```python
from build123d import *

# Parameters (mm, degrees)
SKETCH_W        = 203
SKETCH_H        = 130
SKETCH_R        = 1.75
PAD_DEPTH       = 3
SKETCH001_W     = 4
SKETCH001_H     = 10
PAD001_DEPTH    = 10
SKETCH002_R     = 1.75
SKETCH002_W     = 95
SKETCH002_H     = 4
POCKET_DEPTH    = 225
SKETCH003_R     = 1.75
POCKET001_DEPTH = 200.001


with BuildPart() as part:
    # Sketch → Pad (new body)
    with BuildSketch(Plane.XY):
        with Locations((101.5, 65)):
            Rectangle(SKETCH_W, SKETCH_H)
        with Locations((22, 126.5)):
            Circle(SKETCH_R, mode=Mode.SUBTRACT)
        with Locations((100, 126.5)):
            Circle(SKETCH_R, mode=Mode.SUBTRACT)
        with Locations((178, 126.5)):
            Circle(SKETCH_R, mode=Mode.SUBTRACT)
        with Locations((22, 3.5)):
            Circle(SKETCH_R, mode=Mode.SUBTRACT)
        with Locations((100, 3.5)):
            Circle(SKETCH_R, mode=Mode.SUBTRACT)
        with Locations((178, 3.5)):
            Circle(SKETCH_R, mode=Mode.SUBTRACT)
        with BuildLine():
            ThreePointArc((15, 106.75), (13.25, 105), (15, 103.25))
            Line((15, 103.25), (95, 103.25))
            ThreePointArc((95, 103.25), (96.75, 105), (95, 106.75))
            Line((15, 106.75), (95, 106.75))
        make_face(mode=Mode.SUBTRACT)
        with BuildLine():
            ThreePointArc((14.985188, 96.750011), (13.235188, 95.000011), (14.985188, 93.250011))
            Line((14.985188, 93.250011), (94.985188, 93.250011))
            ThreePointArc((94.985188, 93.250011), (96.735188, 95.000011), (94.985188, 96.750011))
            Line((14.985188, 96.750011), (94.985188, 96.750011))
        make_face(mode=Mode.SUBTRACT)
        with BuildLine():
            ThreePointArc((14.970376, 86.750022), (13.220376, 85.000022), (14.970376, 83.250022))
            Line((14.970376, 83.250022), (94.970376, 83.250022))
            ThreePointArc((94.970376, 83.250022), (96.720376, 85.000022), (94.970376, 86.750022))
            Line((14.970376, 86.750022), (94.970376, 86.750022))
        make_face(mode=Mode.SUBTRACT)
        with BuildLine():
            ThreePointArc((14.955564, 76.750033), (13.205564, 75.000033), (14.955564, 73.250033))
            Line((14.955564, 73.250033), (94.955564, 73.250033))
            ThreePointArc((94.955564, 73.250033), (96.705564, 75.000033), (94.955564, 76.750033))
            Line((14.955564, 76.750033), (94.955564, 76.750033))
        make_face(mode=Mode.SUBTRACT)
        with BuildLine():
            ThreePointArc((14.940752, 66.750044), (13.190752, 65.000044), (14.940752, 63.250044))
            Line((14.940752, 63.250044), (94.940752, 63.250044))
            ThreePointArc((94.940752, 63.250044), (96.690752, 65.000044), (94.940752, 66.750044))
            Line((14.940752, 66.750044), (94.940752, 66.750044))
        make_face(mode=Mode.SUBTRACT)
    extrude(amount=-PAD_DEPTH)

    # Sketch001 (on DatumPlane) → Pad001 (join)
    with BuildSketch(Plane.XY.offset(-3)):
        with Locations((198, 125)):
            Rectangle(SKETCH001_W, SKETCH001_H)
        with Locations((5, 125)):
            Rectangle(SKETCH001_W, SKETCH001_H)
    extrude(amount=-PAD001_DEPTH)

    # Sketch002 → Pocket (cut)
    with BuildSketch(Plane.YZ.offset(107)):
        with Locations((-51, 7)):
            Circle(SKETCH002_R)
        with Locations((61, 7)):
            Circle(SKETCH002_R)
        with Locations((7.5, 11)):
            Rectangle(SKETCH002_W, SKETCH002_H)
    extrude(amount=-POCKET_DEPTH, mode=Mode.SUBTRACT)

    # Sketch003 (on DatumPlane) → Pocket001 (cut, through all)
    with BuildSketch(Plane.YZ.offset(3)):
        with Locations((126.5, -6.5)):
            Circle(SKETCH003_R)
    extrude(amount=POCKET001_DEPTH, mode=Mode.SUBTRACT)


solid = part.part
```
Check sheet for the modelled part. Datum: model origin and axes. Units: mm. A direction names the side the tool comes from. Coordinates: 2 decimals unless noted, no trailing zeros. Order: outer loops, then holes, each group sorted by start corner. A loop starts at its lowest first (then second) coordinate and runs counter-clockwise, first axis right, second up. Notation, with made-up numbers: M -33.75,68.5 L -18.75,68.5 A25 cw -18.75,100.5 Z; hole C 56,74 d8. An arc over 180 degrees is marked long. One line per question, with ' | ' between items. Start each with the question number.
Item 1: Mould release check, pull along X, two halves, no side actions. Record for faces 1 (the flat face through (198, 125, -13)), 2 (the flat face through (7, 125, -8)), 3 (the flat face through (3, 125, -8)): pulls with the +X half, pulls with the -X half, needs draft (parallel to the pull), parting line crosses it, or undercut.
Item 2: Sectioned sample at A-A on x = 27. Record the cut outline in (y, z), and give its area (4 significant figures).
Item 3: Sectioned sample at C-C on x = 105.5. Record the cut outline in (y, z).
Item 4: Access from +Z, -Z, +X, -X, +Y, -Y to the whole of each face (thin tool, end or side, straight path). Record for faces 4 (the flat face through (200, 125, -8)), 5 (the flat face through (198, 120, -8)), 6 (the flat face through (196, 125, -8)), 7 (the flat face through (5, 125, -13)).
Item 5: Gauge pin test, flat ends, axial feed: P1, Ø10, axis at x = 174.5, y = 76, coming from the -Z side; P2, Ø3, axis at y = 126, z = -6.5, coming from the -X side; P3, Ø3, axis at x = 4.5, z = -10, coming from the -Y side. Record the tip position at first contact, or that the pin passes through.
Item 6: Sectioned sample at B-B on y = 27.5. Record the cut outline in (x, z).
Item 7: Material ranges on line 1 (X direction, y = 126.5, z = -2.3); line 2 (Y direction, x = 5.3, z = -6.5); line 3 (Z direction, x = 66.5, y = 44), recorded low to high.
Answer below:
1) face 1: needs draft | face 2: undercut | face 3: pulls with the -X half
2) outline: M 0,-3 L 63.25,-3 L 63.25,0 L 0,0 Z; M 66.75,-3 L 73.25,-3 L 73.25,0 L 66.75,0 Z; M 76.75,-3 L 83.25,-3 L 83.25,0 L 76.75,0 Z; M 86.75,-3 L 93.25,-3 L 93.25,0 L 86.75,0 Z; M 96.75,-3 L 103.25,-3 L 103.25,0 L 96.75,0 Z; M 106.75,-3 L 130,-3 L 130,0 L 106.75,0 Z | area: 337.5 mm^2
3) outline: M 0,-3 L 130,-3 L 130,0 L 0,0 Z
4) face 4: -Z, +X, +Y, -Y | face 5: -Z, +X, -X, -Y | face 6: -Z, +Y, -Y | face 7: -Z, +X, -X, +Y, -Y
5) P1: stops at z = -3 | P2: stops at x = 3 | P3: stops at y = 120
6) outline: M 0,-3 L 203,-3 L 203,0 L 0,0 Z
7) line 1: x = 0 to 20.25, 23.75 to 98.25, 101.75 to 176.25, 179.75 to 203 | line 2: y = 120 to 124.75, 128.25 to 130 | line 3: z = -3 to 0
